from build123d import *

# Parameters (mm, degrees)
SKETCH1_W                = 32.004
SKETCH1_H                = 44.704
BOSS_EXTRUDE1_DEPTH      = 1.5
BOSS_EXTRUDE1_DEPTH_BACK = 0.0254
SKETCH2_W                = 10.668
SKETCH2_H                = 2.54
BOSS_EXTRUDE2_DEPTH      = 2.032
SKETCH4_W                = 10.668
SKETCH4_H                = 1.746
CUT_EXTRUDE1_DEPTH       = 3.81
SKETCH5_W                = 21.844
SKETCH5_H                = 2.54
BOSS_EXTRUDE3_DEPTH      = 3.556
SKETCH10_W               = 33.528
SKETCH10_H               = 46.228
BOSS_EXTRUDE5_DEPTH      = 0.508
SKETCH13_W               = 10.668
SKETCH13_H               = 5.08
CUT_EXTRUDE2_DEPTH       = 8.128


with BuildPart() as part:
    # Sketch1 → Boss-Extrude1 (new body, two sides)
    with BuildSketch(Plane.XY) as boss_extrude1_sk:
        with Locations((12.794077502, 22.352)):
            Rectangle(SKETCH1_W, SKETCH1_H)
    extrude(amount=BOSS_EXTRUDE1_DEPTH)
    extrude(boss_extrude1_sk.sketch, amount=-BOSS_EXTRUDE1_DEPTH_BACK)

    # Sketch2 → Boss-Extrude2 (add)
    with BuildSketch(Plane.XY.offset(1.5)):
        with Locations((12.794077502, 41.434)):
            Rectangle(SKETCH2_W, SKETCH2_H)
    extrude(amount=BOSS_EXTRUDE2_DEPTH)

    # Sketch4 → Cut-Extrude1 (cut)
    with BuildSketch(Plane.XY.offset(1.5)):
        with Locations((12.794077502, 43.831)):
            Rectangle(SKETCH4_W, SKETCH4_H)
    extrude(amount=-CUT_EXTRUDE1_DEPTH, mode=Mode.SUBTRACT)

    # Sketch5 → Boss-Extrude3 (add)
    with BuildSketch(Plane.XY.offset(1.5)):
        with Locations((12.794077502, 1.27)):
            Rectangle(SKETCH5_W, SKETCH5_H)
    extrude(amount=BOSS_EXTRUDE3_DEPTH)

    # Sketch10 → Boss-Extrude5 (add)
    with BuildSketch(Plane(origin=(0, 0, -0.0254), x_dir=(-1, 0, 0), z_dir=(0, 0, -1))):
        with Locations((-12.794077502, 22.352)):
            Rectangle(SKETCH10_W, SKETCH10_H)
    extrude(amount=BOSS_EXTRUDE5_DEPTH)

    # Sketch13 → Cut-Extrude2 (cut)
    with BuildSketch(Plane.XY.offset(3.532)):
        with Locations((12.794077502, 43.974)):
            Rectangle(SKETCH13_W, SKETCH13_H)
    extrude(amount=-CUT_EXTRUDE2_DEPTH, mode=Mode.SUBTRACT)


solid = part.part
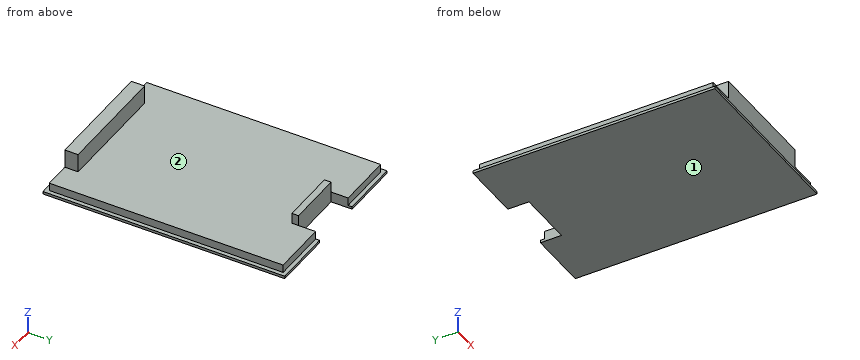
Model file for the job. Use its own axes, mm. Face numbers are marked on the shaded views. Coordinates: 2 decimals unless noted, no trailing zeros. Order: outer loops, then holes, each group sorted by start corner. A loop starts at its lowest first (then second) coordinate and runs counter-clockwise, first axis right, second up. Notation, with made-up numbers: M -26.5,4.5 L 4.5,4.5 A34 ccw 4.5,39.5 Z; hole C 14.25,0 d10. An arc over 180 degrees is marked long. Return JSON: item names as keys, results as strings.
1. Pull direction Y, two halves, no side cores. Call the marked faces 1 and 2: +Y half, -Y half, draft (parallel to the pull), parting line (faces both ways), or undercut.
Ans:
{"face 1": "draft", "face 2": "undercut"}
2. Saw through at D-D (y = 7.5). Give the cut face in (x, z).
Ans:
{"outline": "M -3.97,-0.53 L 29.56,-0.53 L 29.56,-0.03 L 28.8,-0.03 L 28.8,1.5 L -3.21,1.5 L -3.21,-0.03 L -3.97,-0.03 Z"}
3. Saw through at C-C (x = -1). Give the cut face in (y, z), and give its area (3 significant figures).
Ans:
{"outline": "M -0.76,-0.53 L 45.47,-0.53 L 45.47,-0.03 L 44.7,-0.03 L 44.7,1.5 L 0,1.5 L 0,-0.03 L -0.76,-0.03 Z", "area": "91.7 mm^2"}
4. Saw through at A-A (z = 3.05). Give the cut face in (x, y).
Ans:
{"outline": "M 1.87,0 L 23.72,0 L 23.72,2.54 L 1.87,2.54 Z; M 7.46,40.16 L 18.13,40.16 L 18.13,41.43 L 7.46,41.43 Z"}
5. Drill centre lines: probe 1 along Y at (x, z) = (13.5, 3.15); probe 2 along Y at (x, z) = (5.5, 4.1); probe 3 along X at (y, z) = (1, 0.1). Where is each one in solid material? Low to high.
Ans:
{"probe 1": "0 to 2.54, 40.16 to 41.43", "probe 2": "0 to 2.54", "probe 3": "-3.21 to 28.8"}
6. Saw through at B-B (y = 42.5). Give the cut face in (x, z), and give its area (3 significant figures).
Ans:
{"outline": "M -3.97,-0.53 L 7.46,-0.53 L 7.46,1.5 L -3.21,1.5 L -3.21,-0.03 L -3.97,-0.03 Z; M 18.13,-0.53 L 29.56,-0.53 L 29.56,-0.03 L 28.8,-0.03 L 28.8,1.5 L 18.13,1.5 Z", "area": "44.2 mm^2"}
7. Flat gauge pins, fed straight in: pin 1 (1.5 mm diameter, centred on x = 14.5, y = 10, fed in from +Z); pin 2 (2 mm diameter, centred on x = 6, z = 4.5, fed in from -Y); pin 3 (2 mm diameter, centred on y = 44.5, z = 0.5, fed in from -X); pin 4 (0.5 mm diameter, centred on y = 22, z = 0.5, fed in from -X). Where does each tip first touch, or does it go through?
Ans:
{"pin 1": "z = 1.5", "pin 2": "y = 0", "pin 3": "x = -3.97", "pin 4": "x = -3.21"}
